Input: dimensioned drawing with shaded views. Units: mm. Origin: part minimum x, y, z. A direction names the side the tool comes from. Round coordinates to 2 decimals unless told otherwise and drop trailing zeros. Write each loop counter-clockwise with the first axis right and the second up, starting at its lowest first coordinate (ties: lowest second). Pieces come first, ordered by that corner, then holes. Notation, with made-up numbers: (-15.75, -40) - (9.25, -40) arc R14 ccw to (9.25, -33) - close; hole circle Ø6 at (-9, 44.5). An arc over 180 degrees is marked (long way). Use one line per item in the form item = value.
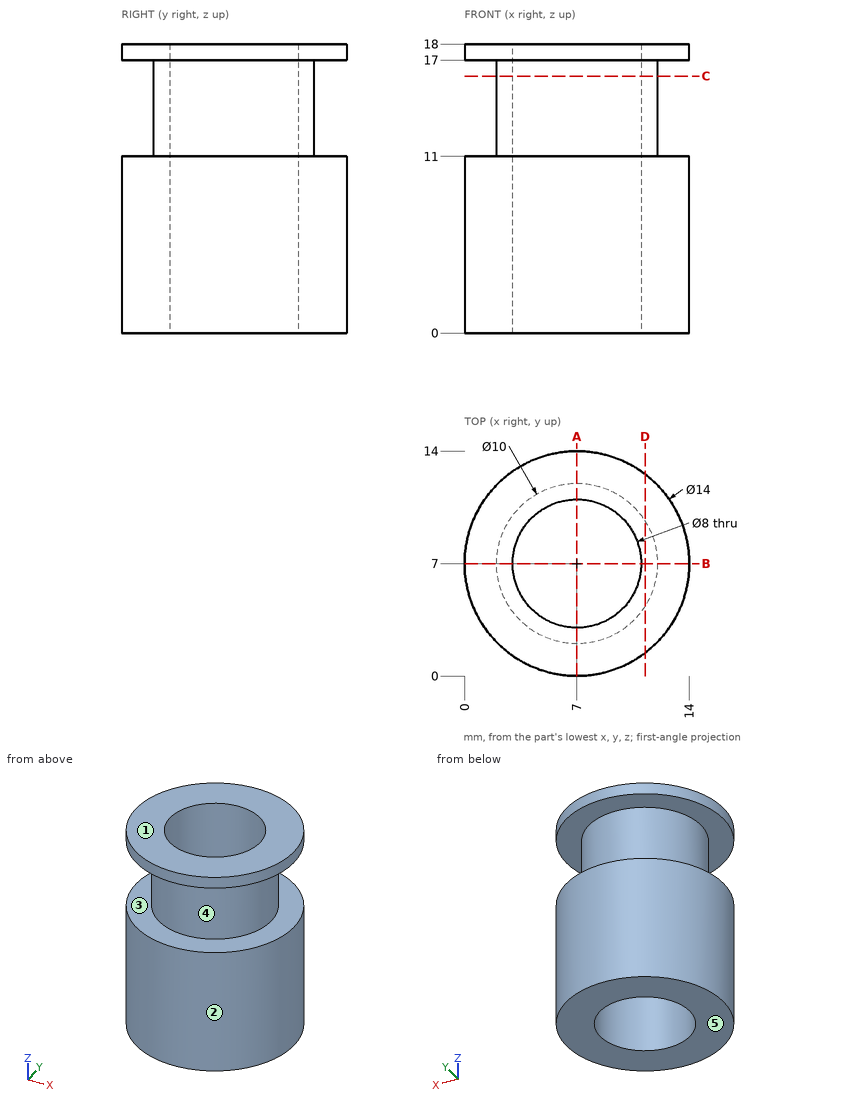
(1) Access query for the marked faces 4 and 5. Directions: +Z, -Z, +X, -X, +Y, -Y. A direction counts if a zero-diameter tool reaches every point of the face in a straight line with its end or side. Return the directions, or none.
Derived:
face_4 = none
face_5 = -Z, +X, -X, +Y, -Y
(2) Cut plane D-D on x = 11.25. Output: boundary loops of the cut face in (y, z).
Derived:
outline = (1.44, 0) - (12.56, 0) - (12.56, 11) - (9.63, 11) - (9.63, 17) - (12.56, 17) - (12.56, 18) - (1.44, 18) - (1.44, 17) - (4.37, 17) - (4.37, 11) - (1.44, 11) - close
(3) First-contact query: pin 1 Ø1 at (y, z) = (10.5, 15) entering from -X; pin 2 Ø1 at (y, z) = (6, 8) entering from +X; pin 3 Ø1 at (y, z) = (12.5, 7.5) entering from +X. Flat tips, straight axial feed; report the tip coordinate or a pass-through.
Derived:
pin_1 = 3
pin_2 = 13.98
pin_3 = 11.9
(4) Draft query along Z for the marked faces 1, 2 and 3. Return one class per face: released by +Z, released by -Z, zero draft, split by the parting line, or undercut.
Derived:
face_1 = released by +Z
face_2 = zero draft
face_3 = undercut
(5) Material intervals for L1, parallel to Z at x = 2.5, y = 2; L2, parallel to Y at x = 7, z = 5.75; L3, parallel to Y at x = 9.5, z = 8.75, sorted ascending.
Derived:
L1 = 0 to 11, 17 to 18
L2 = 0 to 3, 11 to 14
L3 = 0.46 to 3.88, 10.12 to 13.54
(6) Cut plane C-C on z = 16. Output: boundary loops of the cut face in (x, y), then the cut area to 3 significant figures.
Derived:
outline = circle Ø10 at (7, 7); hole circle Ø8 at (7, 7)
area = 28.3 mm^2
(7) Cut plane A-A on x = 7. Output: boundary loops of the cut face in (y, z), then the cut area to 3 significant figures.
Derived:
outline = (0, 0) - (3, 0) - (3, 18) - (0, 18) - (0, 17) - (2, 17) - (2, 11) - (0, 11) - close; (11, 0) - (14, 0) - (14, 11) - (12, 11) - (12, 17) - (14, 17) - (14, 18) - (11, 18) - close
area = 84.0 mm^2
